Part model, mm, in its own coordinate system. Round coordinates to 2 decimals unless told otherwise and drop trailing zeros. Write each loop counter-clockwise with the first axis right and the second up, starting at its lowest first coordinate (ties: lowest second). Pieces come first, ordered by that corner, then holes. Notation, with made-up numbers: M 36,-9.5 L 69,-9.5 A30 ccw 69,21.5 Z; hole C -9,27 d10. An arc over 180 degrees is marked long. Answer as a JSON object with one key per item and string values. Group by question number.
1. Band-saw the part on B-B, the plane y = 0. Write the cut outline in (x, z).
2. Two-plate mould, pull along Z, no slides. Class faces 1 (the face through (6, -126, -49.483)), 2 (the face through (12.7, -126, 60)), 3 (the face through (6.26, -1.72, -19.13)), 4 (the face through (6, -126, 166.417)): +Z half, -Z half, draft (parallel to the pull), parting line (faces both ways), or undercut.
3. Drill centre lines: line 1 (Z direction, x = 8.5, y = -444.5); line 2 (Y direction, x = 6, z = -24); line 3 (Y direction, x = 10.75, z = -18.5). Where is each one in solid material? Low to high. Write a range as from..to.
4. Band-saw the part on A-A, the plane y = -444.5. Write the cut outline in (x, z), plus the area to 3 significant figures.
from build123d import *

# Parameters (mm, degrees)
F0_W     = 698.5
F0_H     = 215.9
F0_R     = 6.35
F0_R_2   = 7.9375
F1_DEPTH = 12.7


with BuildPart() as f1:
    # F0 (on Right) → F1 (new body)
    with BuildSketch(Plane.YZ):
        with Locations((-120.65, 58.467444)):
            Rectangle(F0_W, F0_H)
        with Locations((-444.5, -24.082556)):
            Circle(F0_R, mode=Mode.SUBTRACT)
        with Locations((0, -11.382556)):
            Circle(F0_R_2, mode=Mode.SUBTRACT)
        with Locations((-444.5, 141.017444)):
            Circle(F0_R, mode=Mode.SUBTRACT)
    extrude(amount=F1_DEPTH)


solid = f1.part
Worked answers:
{
 "1": {"outline": "M 0,-49.48 L 12.7,-49.48 L 12.7,-19.32 L 0,-19.32 Z; M 0,-3.45 L 12.7,-3.45 L 12.7,166.42 L 0,166.42 Z"},
 "2": {"face 1": "-Z half", "face 2": "draft", "face 3": "undercut", "face 4": "+Z half"},
 "3": {"line 1": "z = -49.48..-30.43, -17.73..134.67, 147.37..166.42", "line 2": "y = -469.9..-450.85, -438.15..228.6", "line 3": "y = -469.9..-447.53, -441.47..-3.51, 3.51..228.6"},
 "4": {"outline": "M 0,-49.48 L 12.7,-49.48 L 12.7,-30.43 L 0,-30.43 Z; M 0,-17.73 L 12.7,-17.73 L 12.7,134.67 L 0,134.67 Z; M 0,147.37 L 12.7,147.37 L 12.7,166.42 L 0,166.42 Z", "area": "2,420 mm^2"}
}
